The model under review builds one solid part; all positions refer to its coordinate system, in mm. A direction names the side the tool comes from. Round coordinates to 2 decimals unless told otherwise and drop trailing zeros. Loops run counter-clockwise (first coordinate to the right, second up) from the corner with the lowest first, then second, coordinate; pieces in that order, holes last. Notation, with made-up numbers: (-11, -31) -> (13, -31) arc R18 cw to (13, -26) -> close; hole circle Ø2 at (-26.75, 26). An arc over 180 degrees is marked (long way). Use a Markdown table: item, result. Add a question column.
1) Mouldability with a two-part tool opening along X and no side actions: class faces 5 (the flat face through (4, 6, 3.256)), 6 (the flat face through (116.84, 1, 16)), 7 (the flat face through (95.657, 6, 10)) as released by +X, released by -X, zero draft, split by the parting line, or undercut.
2) Insertion check: pin 1 (3 mm diameter, centred on y = 4.5, z = 7, fed in from +X); pin 2 (2 mm diameter, centred on y = 5, z = 23.5, fed in from +X); pin 3 (4.5 mm diameter, centred on x = 63, z = 23.5, fed in from +Y). Each pin has a flat end and moves straight along its axis. Give the tip position at first contact, or say it passes through.
3) For faces 1 (the flat face through (106, 2.54, 14)), 2 (the flat face through (35, 6, 18.317)), 3 (the flat face through (25.096, 5.671, 26.591)), 4 (the flat face through (17.096, 6, 2)), list the 3-axis set-ups (+Z, -Z, +X, -X, +Y, -Y) from which the entire face can be reached by the end or side of a thin tool; tool diameter is ignored.
4) Wall thickness on probe 1 along Z at (x, y) = (12, 1.5); probe 2 along Y at (x, z) = (46, 11); probe 3 along X at (y, z) = (2.75, 3.5): over which ranges is each line inside the solid? List them lowest first.
5) Consider section A-A on y = 1.25. Give the boundary of the cut face in (x, z), plus the area to 3 significant figures.
6) Consider section B-B on x = 44. Give the boundary of the cut face in (y, z).
from build123d import *

# Parameters (mm, degrees)
SKETCH2_W           = 116.84
SKETCH2_H           = 31.75
BOSS_EXTRUDE2_DEPTH = 2.54
BOSS_EXTRUDE5_DEPTH = 6.35


with BuildPart() as part:
    # Sketch2 → Boss-Extrude2 (new body)
    with BuildSketch(Plane(origin=(0, 0, 0), x_dir=(1, 0, 0), z_dir=(0, 1, 0))):
        with Locations((58.42, -15.875)):
            Rectangle(SKETCH2_W, SKETCH2_H)
    extrude(amount=BOSS_EXTRUDE2_DEPTH)

    # Sketch6 → Boss-Extrude5 (add)
    # profile 1 of 4: a face of its own
    with BuildSketch(Plane(origin=(0, 2.54, 0), x_dir=(1, 0, 0), z_dir=(0, 1, 0))):
        Polygon((0.407051282, -3.256410256), (0.407051282, 0), (17.096153846, 0), (17.096153846, -3.256410256), (10.176282051, -3.256410256), (10.176282051, -31.75), (7.326923077, -31.75), (7.326923077, -3.256410256), align=None)
    # profile 2 of 4: a face of its own
    with BuildSketch(Plane(origin=(0, 2.54, 0), x_dir=(1, 0, 0), z_dir=(0, 1, 0))):
        Polygon((35.006410256, 0), (49.66025641, -31.75), (46.562850561, -31.75), (41.869040465, -21.573717949), (27.475961538, -21.573717949), (22.64858774, -31.75), (19.538461538, -31.75), (34.599358974, 0), align=None)
        Polygon((34.771083734, -6.188451522), (29.021484375, -18.317307692), (40.368038862, -18.317307692), align=None, mode=Mode.SUBTRACT)
    # profile 3 of 4: a face of its own
    with BuildSketch(Plane(origin=(0, 2.54, 0), x_dir=(1, 0, 0), z_dir=(0, 1, 0))):
        Polygon((53.730769231, -31.75), (57.922125401, 0), (58.329176683, 0), (71.4375, -26.051282051), (84.514022436, 0), (84.927433894, 0), (89.144230769, -31.75), (86.282151442, -31.75), (83.241987179, -8.904246795), (71.780949519, -31.75), (71.138571715, -31.75), (59.633012821, -8.853365385), (56.599208734, -31.75), align=None)
    # profile 4 of 4: a face of its own
    with BuildSketch(Plane(origin=(0, 2.54, 0), x_dir=(1, 0, 0), z_dir=(0, 1, 0))):
        with BuildLine():
            Line((95.657051282, 0), (98.506410256, 0))
            Line((98.506410256, 0), (98.506410256, -19.02328726))
            add(Edge.make_bspline(
                [(98.506410256, -19.02328726), (98.505986222, -19.292533934), (98.505181543, -19.803475897), (98.51055649, -20.530716909), (98.525609332, -21.177259931), (98.535099494, -21.745597155), (98.556211734, -22.23312065), (98.573429731, -22.642471683), (98.595569067, -22.971711948), (98.622176633, -23.163853206), (98.633613782, -23.246444311)],
                knots=[0, 0, 0, 0, 1.528628734, 2.90083645, 4.128790002, 5.200304208, 6.127813768, 6.898992206, 7.526736466, 8, 8, 8, 8], degree=3))
            add(Edge.make_bspline(
                [(98.633613782, -23.246444311), (98.68058073, -23.544411378), (98.771868206, -24.123556136), (99.00451749, -24.948224121), (99.329433392, -25.691459492), (99.714452422, -26.376454776), (100.221841111, -26.984143971), (100.829658895, -27.543956821), (101.566057224, -28.033558192), (102.384849861, -28.481240556), (103.267365944, -28.841059518), (104.169168146, -29.11314218), (105.076700886, -29.278957914), (105.684270383, -29.298157946), (105.985977564, -29.307692308)],
                knots=[0, 0, 0, 0, 1.035780045, 2.013197591, 2.933192213, 3.817615948, 4.702609284, 5.640816605, 6.646850145, 7.73207398, 8.84249596, 9.914020372, 10.964143139, 12, 12, 12, 12], degree=3))
            add(Edge.make_bspline(
                [(105.985977564, -29.307692308), (106.245000781, -29.297950952), (106.761551163, -29.278524503), (107.529052356, -29.158224378), (108.276539056, -28.941412104), (109.007702367, -28.661651438), (109.693057725, -28.292012576), (110.332987521, -27.865012818), (110.904160353, -27.3641713), (111.425386476, -26.809903889), (111.879274822, -26.184521418), (112.272713036, -25.501641166), (112.594983969, -24.750986376), (112.754128801, -24.223442688), (112.83588742, -23.952423878)],
                knots=[0, 0, 0, 0, 0.994687771, 1.983630487, 2.973142513, 3.978332533, 4.983357753, 5.956394766, 6.925816176, 7.893390482, 8.871859704, 9.88551698, 10.913711441, 12, 12, 12, 12], degree=3))
            add(Edge.make_bspline(
                [(112.83588742, -23.952423878), (112.863102842, -23.840404668), (112.923749771, -23.590780724), (112.980419393, -23.16876616), (113.039442874, -22.670841216), (113.080396473, -22.093428342), (113.12032183, -21.438462376), (113.144207562, -20.702531326), (113.155247789, -19.888307468), (113.158537818, -19.320098929), (113.16025641, -19.02328726)],
                knots=[0, 0, 0, 0, 0.558680831, 1.244966039, 2.062412453, 2.990489873, 4.051219941, 5.244515665, 6.560634259, 8, 8, 8, 8], degree=3))
            Line((113.16025641, -19.02328726), (113.16025641, 0))
            Line((113.16025641, 0), (116.009615385, 0))
            Line((116.009615385, 0), (116.009615385, -19.17593149))
            add(Edge.make_bspline(
                [(116.009615385, -19.17593149), (116.00731015, -19.521538214), (116.002811344, -20.196010747), (115.963798971, -21.184355218), (115.901596187, -22.121914406), (115.813711389, -23.008814339), (115.697261431, -23.841881355), (115.567764788, -24.628417466), (115.402850453, -25.362776756), (115.21023317, -26.050685116), (114.990037413, -26.705510845), (114.704821282, -27.32698185), (114.383470461, -27.933991046), (114.002337538, -28.517357463), (113.574062853, -29.079664052), (113.089179749, -29.617500661), (112.563724861, -30.139462009), (111.988963142, -30.632159109), (111.374369091, -31.083994964), (110.721770904, -31.481303316), (110.036181635, -31.817160417), (109.31938342, -32.093620589), (108.571070365, -32.301488739), (107.791223602, -32.456384795), (106.978068062, -32.544398494), (106.425031538, -32.557478859), (106.144981971, -32.564102564)],
                knots=[0, 0, 0, 0, 1.316592851, 2.569410997, 3.76748051, 4.895814652, 5.963796859, 6.97159953, 7.931736103, 8.829262218, 9.692595152, 10.560224239, 11.431080259, 12.30701507, 13.211635791, 14.121146779, 15.063487852, 16.031507147, 17.00238618, 17.966455255, 18.938106653, 19.907068911, 20.888905087, 21.893141452, 22.933117798, 24, 24, 24, 24], degree=3))
            add(Edge.make_bspline(
                [(106.144981971, -32.564102564), (105.839555112, -32.556983622), (105.240308706, -32.543016283), (104.357313382, -32.462981336), (103.510820315, -32.312228759), (102.691889145, -32.120277841), (101.911669207, -31.855539652), (101.159707247, -31.546220948), (100.448882068, -31.166334373), (99.767661973, -30.743665736), (99.134251685, -30.268099376), (98.552796671, -29.749756369), (98.022336988, -29.196940088), (97.551813814, -28.603665342), (97.133431504, -27.974546285), (96.773021711, -27.307803182), (96.463565853, -26.603694171), (96.303849138, -26.114261567), (96.223106971, -25.866836939)],
                knots=[0, 0, 0, 0, 1.13879206, 2.234305948, 3.301075583, 4.341971843, 5.366689343, 6.369221514, 7.369726634, 8.367512178, 9.355451585, 10.318319045, 11.268648973, 12.207971039, 13.137398894, 14.081662264, 15.030215811, 16, 16, 16, 16], degree=3))
            add(Edge.make_bspline(
                [(96.223106971, -25.866836939), (96.176142751, -25.697812871), (96.07427631, -25.331195903), (95.965189682, -24.724439899), (95.87348587, -24.025804575), (95.787256877, -23.235242108), (95.736375616, -22.352139747), (95.691767422, -21.376880296), (95.656737023, -20.308284501), (95.656943601, -19.563932823), (95.657051282, -19.17593149)],
                knots=[0, 0, 0, 0, 0.625038921, 1.35572334, 2.194682327, 3.136881307, 4.189498639, 5.346923369, 6.617055217, 8, 8, 8, 8], degree=3))
            Line((95.657051282, -19.17593149), (95.657051282, 0))
        make_face()
    extrude(amount=BOSS_EXTRUDE5_DEPTH)


solid = part.part
Result set:
| question | item | result |
|---|---|---|
| 1 | face 5 | zero draft |
| 1 | face 6 | released by +X |
| 1 | face 7 | undercut |
| 2 | pin 1 | x = 116.01 |
| 2 | pin 2 | x = 115.86 |
| 2 | pin 3 | y = 2.54 |
| 3 | face 1 | -Z, +Y |
| 3 | face 2 | +Y |
| 3 | face 3 | +Z, +Y |
| 3 | face 4 | +Z, -Z, +Y |
| 4 | probe 1 | 0 to 31.75 |
| 4 | probe 2 | 0 to 2.54 |
| 4 | probe 3 | 7.33 to 10.18, 32.94 to 36.62, 57.46 to 60.09, 82.76 to 85.39, 95.66 to 98.51, 113.16 to 116.01 |
| 5 | outline | (0, 0) -> (116.84, 0) -> (116.84, 31.75) -> (0, 31.75) -> close |
| 5 | area | 3,710 mm2 |
| 6 | outline | (0, 0) -> (2.54, 0) -> (2.54, 19.49) -> (8.89, 19.49) -> (8.89, 26.19) -> (2.54, 26.19) -> (2.54, 31.75) -> (0, 31.75) -> close |
